from build123d import *

# Parameters (mm, degrees)
F0_W        = 88.9
F0_H        = 165.1
F1_DEPTH    = 6.35
F2_DEPTH    = 25.4
F3_SIZE     = 5.08
F4_DEPTH    = 50.8
F5_R        = 5.08
F6_C1_SIZE2 = 12.7
F6_C1_SIZE  = 7.3323484187
F6_C2_SIZE2 = 7.3323484187
F6_C2_SIZE  = 12.7
F6_C3_SIZE2 = 7.3323484187
F6_C3_SIZE  = 12.7
F6_C4_SIZE2 = 7.3323484187
F6_C4_SIZE  = 12.7


with BuildPart() as f1:
    # F0 (on Top) → F1 (new body)
    with BuildSketch(Plane.XY):
        Rectangle(F0_W, F0_H)
        Polygon((-38.1, 38.1), (-38.1, 76.2), (0, 76.2), (38.1, 76.2), (38.1, -38.1), (38.1, -76.2), (0, -76.2), (-38.1, -76.2), align=None, mode=Mode.SUBTRACT)
    extrude(amount=F1_DEPTH)

    # F0 (on Top) → F2 (join)
    with BuildSketch(Plane.XY):
        with BuildLine():
            Line((38.1, 76.2), (0, 76.2))
            Line((0, 76.2), (0, 50.8))
            ThreePointArc((0, 50.8), (-3.7197438789, 41.8197438789), (-12.7, 38.1))
            Line((-12.7, 38.1), (-38.1, 38.1))
            Line((-38.1, 38.1), (-38.1, -76.2))
            Line((-38.1, -76.2), (0, -76.2))
            Line((0, -76.2), (0, -50.8))
            ThreePointArc((0, -50.8), (3.7197438789, -41.8197438789), (12.7, -38.1))
            Line((12.7, -38.1), (38.1, -38.1))
            Line((38.1, -38.1), (38.1, 76.2))
        make_face()
    extrude(amount=F2_DEPTH)

    # F3
    f3_edges = [f1.edges().sort_by_distance(p)[0] for p in [
        (-38.1, -19.05, 25.4),
        (-19.05, -76.2, 25.4),
        (38.1, 19.05, 25.4),
        (19.05, 76.2, 25.4),
    ]]
    chamfer(f3_edges, length=F3_SIZE)

    # F0 (on Top) → F4 (join)
    with BuildSketch(Plane.XY):
        with BuildLine():
            Line((38.1, -76.2), (38.1, -38.1))
            Line((38.1, -38.1), (12.7, -38.1))
            ThreePointArc((12.7, -38.1), (3.7197438789, -41.8197438789), (0, -50.8))
            Line((0, -50.8), (0, -76.2))
            Line((0, -76.2), (38.1, -76.2))
        make_face()
        with BuildLine():
            Line((0, 76.2), (-38.1, 76.2))
            Line((-38.1, 76.2), (-38.1, 38.1))
            Line((-38.1, 38.1), (-12.7, 38.1))
            ThreePointArc((-12.7, 38.1), (-3.7197438789, 41.8197438789), (0, 50.8))
            Line((0, 50.8), (0, 76.2))
        make_face()
    extrude(amount=F4_DEPTH)

    # F5
    f5_edges = [f1.edges().sort_by_distance(p)[0] for p in [
        (0, 82.55, 6.35),
        (-44.45, 0, 6.35),
        (0, -82.55, 6.35),
        (44.45, 0, 6.35),
    ]]
    fillet(f5_edges, radius=F5_R)

    # F6: chamfer of 12.7 x 7.3323484187 on 4 edges, made by hand

    # F6_c1
    f6_c1_edges = [f1.edges().sort_by_distance(p)[0] for p in [
        (-38.1, 57.15, 50.8),
    ]]
    f6_c1_side = f1.faces().sort_by_distance((-38.1, 57.15, 50.6533530316))[0]
    chamfer(f6_c1_edges, length=F6_C1_SIZE, length2=F6_C1_SIZE2, reference=f6_c1_side)

    # F6_c2
    f6_c2_edges = [f1.edges().sort_by_distance(p)[0] for p in [
        (-12.7, 76.2, 50.8),
    ]]
    f6_c2_side = f1.faces().sort_by_distance((-12.7, 76.2, 50.6533530316))[0]
    chamfer(f6_c2_edges, length=F6_C2_SIZE, length2=F6_C2_SIZE2, reference=f6_c2_side)

    # F6_c3
    f6_c3_edges = [f1.edges().sort_by_distance(p)[0] for p in [
        (38.1, -57.15, 50.8),
    ]]
    f6_c3_side = f1.faces().sort_by_distance((38.1, -57.15, 50.6533530316))[0]
    chamfer(f6_c3_edges, length=F6_C3_SIZE, length2=F6_C3_SIZE2, reference=f6_c3_side)

    # F6_c4
    f6_c4_edges = [f1.edges().sort_by_distance(p)[0] for p in [
        (15.3838257906, -76.2, 50.8),
    ]]
    f6_c4_side = f1.faces().sort_by_distance((15.3838257906, -76.2, 50.6533530316))[0]
    chamfer(f6_c4_edges, length=F6_C4_SIZE, length2=F6_C4_SIZE2, reference=f6_c4_side)


solid = f1.part
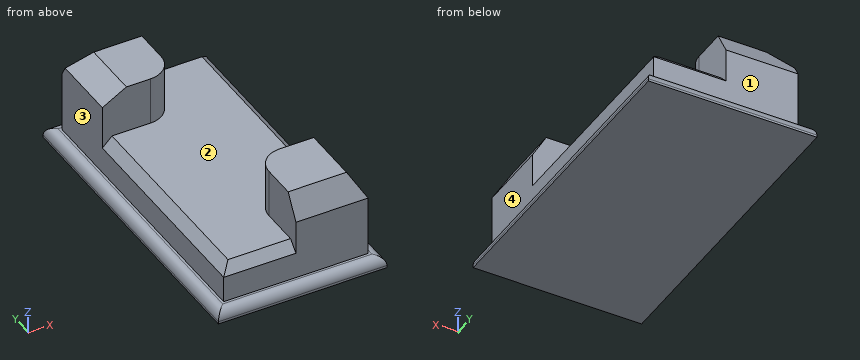
Work out the finished part from the listing and answer in its coordinate system (mm). Face numbers are marked on the shaded views. A direction names the side the tool comes from. Round coordinates to 2 decimals unless told otherwise and drop trailing zeros. Loops run counter-clockwise (first coordinate to the right, second up) from the corner with the lowest first, then second, coordinate; pieces in that order, holes last. Notation, with made-up numbers: (34, -8.5) - (63, -8.5) arc R25 ccw to (63, 19.5) - close; hole circle Ø7 at (-32, 16.25). An arc over 180 degrees is marked (long way). Use one line per item in the form item = value. Start each with the question number.
(1) Which of the six approach directions +Z, -Z, +X, -X, +Y, -Y give full straight-line access (tool end or side, diameter ignored) to the marked faces 1, 2, 3 and 4?
(2) Find section C-C on x = -20.5. Determine the outline of the cut face in (y, z), and give its area (3 significant figures).
(3) Flat-ended cylindrical pins translate along their axes: P1, Ø12, axis at x = 6.5, z = 26.5, coming from the +Y side; P2, Ø9.5, axis at x = 3, z = 25.5, coming from the +Y side; P3, Ø12.5, axis at y = 62, z = 42, coming from the +X side. Find the tip coordinate at first contact, or state that the pin passes through.
(4) Find section A-A on z = 32.5. Determine the outline of the cut face in (x, y).
(5) Find section B-B on y = 65. Determine the outline of the cut face in (x, z).
(6) Find section D-D on z = 12. Determine the outline of the cut face in (x, y).
(7) Consider line 1 (Y direction, x = -6, z = 12.5); line 2 (Z direction, x = -18.5, y = -36); line 3 (X direction, y = 18.5, z = 10.5). Determine where each line is inside the solid, lowest interval first.
Answer list:
q1.face_1 = +Z, +X, -X, +Y
q1.face_2 = +Z
q1.face_3 = +Z, -X, +Y, -Y
q1.face_4 = +Z, +X, +Y, -Y
q2.outline = (-82.55, 0) - (82.55, 0) - (82.55, 1.27) arc R5.08 ccw to (77.47, 6.35) - (76.2, 6.35) - (76.2, 38.1) - (68.87, 50.8) - (38.1, 50.8) - (38.1, 25.4) - (-71.12, 25.4) - (-76.2, 20.32) - (-76.2, 6.35) - (-77.47, 6.35) arc R5.08 ccw to (-82.55, 1.27) - close
q2.area = 4,850 mm^2
q3.P1 = 76.02
q3.P2 = 76.2
q3.P3 = 0
q4.outline = (-38.1, 38.1) - (-12.7, 38.1) arc R12.7 ccw to (0, 50.8) - (0, 76.2) - (-38.1, 76.2) - close; (0, -76.2) - (38.1, -76.2) - (38.1, -38.1) - (12.7, -38.1) arc R12.7 ccw to (0, -50.8) - close
q5.outline = (-44.45, 0) - (44.45, 0) - (44.45, 1.27) arc R5.08 ccw to (39.37, 6.35) - (38.1, 6.35) - (38.1, 20.32) - (33.02, 25.4) - (0, 25.4) - (0, 50.8) - (-25.4, 50.8) - (-38.1, 43.47) - (-38.1, 6.35) - (-39.37, 6.35) arc R5.08 ccw to (-44.45, 1.27) - close
q6.outline = (-38.1, -76.2) - (38.1, -76.2) - (38.1, 76.2) - (-38.1, 76.2) - close
q7.line_1 = -76.2 to 76.2
q7.line_2 = 0 to 25.4
q7.line_3 = -38.1 to 38.1
